Could you check a few things on this drawing? It's one solid part, dimensions in mm from its lowest x, y, z. Give positions to 0.01 mm unless a question says otherwise; leave off trailing zeros. Order: outer loops, then holes, each group sorted by start corner. A loop starts at its lowest first (then second) coordinate and runs counter-clockwise, first axis right, second up.
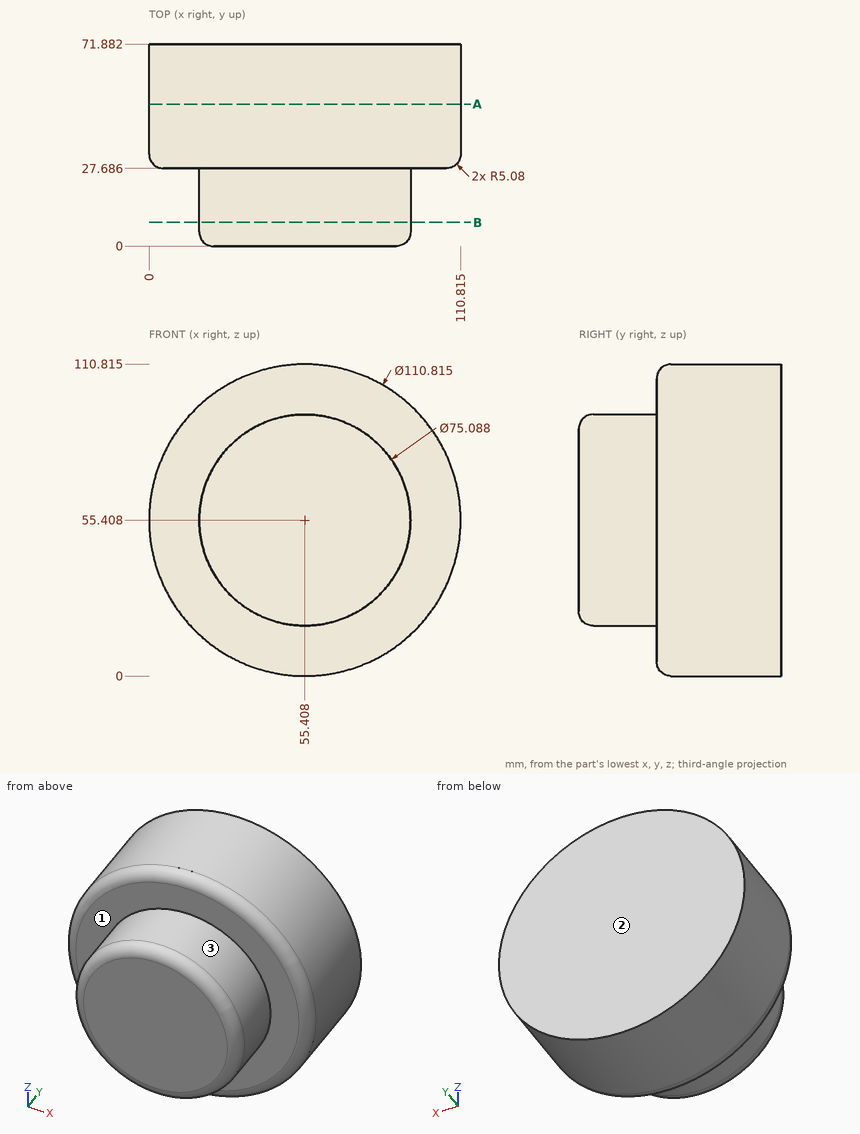
Item 1: For pin 1 (8 mm diameter, centred on x = 22, y = 10, fed in from -Z); pin 2 (4 mm diameter, centred on x = 51.5, y = 49, fed in from -Z); pin 3 (1.5 mm diameter, centred on y = 10, z = 69, fed in from +X), each with a flat end and sliding along its axis, tell me the tip position at first contact or that it passes through.
Findings:
pin 1: stops at z = 32.07
pin 2: stops at z = 0.03
pin 3: stops at x = 90.69
Item 2: Imagine slicing it at B-B on y = 8.5. List the corners of the cut face in (x, z) for me.
Findings:
outline: circle Ø75.09 at (55.41, 55.41)
Item 3: Please list where these lines run through material, in increasing order: line 1 along Y through (x, z) = (13, 55.5); line 2 along Y through (x, z) = (88, 55); line 3 along X through (y, z) = (53, 56).
Findings:
line 1: y = 27.69 to 71.88
line 2: y = 0 to 71.88
line 3: x = 0 to 110.81
Item 4: Imagine slicing it at A-A on y = 50.5. List the corners of the cut face in (x, z) for me (1 decimal).
Findings:
outline: circle Ø110.8 at (55.4, 55.4)
Item 5: We'd pull the mould along Y, two halves only. Please class the marked faces 1, 2 and 3: +Y half, -Y half, draft (parallel to the pull), parting line (faces both ways), or undercut.
Findings:
face 1: -Y half
face 2: +Y half
face 3: draft
